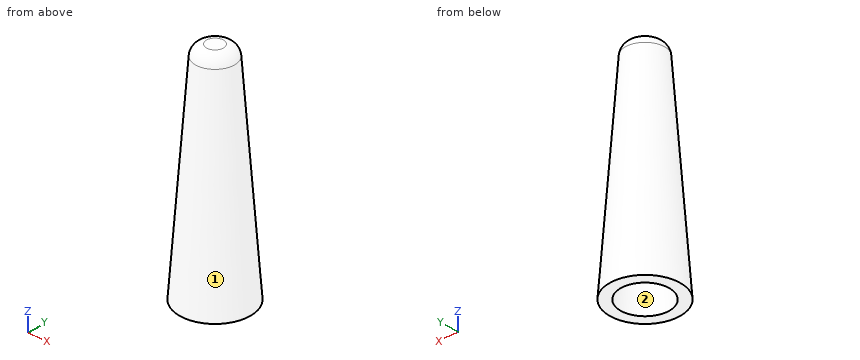
from build123d import *

# Parameters (mm, degrees)
F0_R = 3.2
F2_R = 1.7
F4_T = -1
F5_R = 1


with BuildPart() as f3:
    # F0 (on Top) → F3 section 0
    with BuildSketch(Plane.XY):
        Circle(F0_R)
    # F2 (on offset) → F3 section 1
    with BuildSketch(Plane.XY.offset(20)):
        Circle(F2_R)
    loft()

    # F4
    f4_openings = [f3.faces().sort_by_distance(p)[0] for p in [
        (0, 0, 0),
    ]]
    offset(amount=F4_T, openings=f4_openings, kind=Kind.INTERSECTION)

    # F5
    f5_edges = [f3.edges().sort_by_distance(p)[0] for p in [
        (-1.7, 0, 20),
    ]]
    fillet(f5_edges, radius=F5_R)


solid = f3.part
For this review, take the finished solid that the model builds, in its own axes (mm). Face numbers are marked on the shaded views. Give positions to 0.01 mm unless a question says otherwise; leave off trailing zeros. Loops run counter-clockwise (first coordinate to the right, second up) from the corner with the lowest first, then second, coordinate; pieces in that order, holes last. Notation, with made-up numbers: M 74,-12.5 L 104,-12.5 A5 ccw 104,-3.5 Z; hole C 46,74 d4. An arc over 180 degrees is marked long. Put each result on its own line as item: value. Start each with the question number.
(1) For pin 1 (0.5 mm diameter, centred on x = 0, y = 0, fed in from -Z); pin 2 (2 mm diameter, centred on x = -2.5, z = 8, fed in from -Y); pin 3 (3 mm diameter, centred on x = 2.5, z = 7, fed in from +Y), all flat-tipped, find the tip position at first contact; note any pin that passes through.
(2) The part is to be moulded in two halves that separate along Y. For the marked faces 1 and 2, say which applies: +Y half, -Y half, draft (parallel to the pull), parting line (faces both ways), or undercut.
(3) Add section B-B, the plane z = 5.25. Write out the cut boundary in (x, y), then the cut area to 3 significant figures.
(4) Add section A-A, the plane z = 14.5. Write out the cut boundary in (x, y) (1 decimal), then the cut area to 3 significant figures.
(5) Wall thickness on L1, parallel to Y at x = -0.25, z = 5.25; L2, parallel to Y at x = 0, z = 13 (3 decimals); L3, parallel to X at y = -0.25, z = 7: over which ranges is each line inside the solid? List them lowest first.
Result:
1. pin 1: stops at z = 19
1. pin 2: stops at y = -2.13
1. pin 3: stops at y = 2.49
2. face 1: parting line
2. face 2: undercut
3. outline: C 0,0 d5.61; hole C 0,0 d3.61
3. area: 14.5 mm^2
4. outline: C 0,0 d4.2; hole C 0,0 d2.2
4. area: 10.2 mm^2
5. L1: y = -2.8 to -1.79, 1.79 to 2.8
5. L2: y = -2.225 to -1.222, 1.222 to 2.225
5. L3: x = -2.66 to -1.65, 1.65 to 2.66
